Model file for the job. Use its own axes, mm. Round coordinates to 2 decimals unless told otherwise and drop trailing zeros. Order: outer loops, then holes, each group sorted by start corner. A loop starts at its lowest first (then second) coordinate and runs counter-clockwise, first axis right, second up. Notation, with made-up numbers: (60, -2.75) - (79, -2.75) arc R9 cw to (79, 1.25) - close; hole circle Ø4 at (62, 83.25). An arc over 180 degrees is marked (long way). Put each result on its own line as item: value. Start each with the question number.
Item 1: Saw through at A-A on z = 41. List the corners of the cut face in (x, y).
Item 2: Probe probe 1 along Y at (x, z) = (36.5, 70); probe 2 along Z at (x, y) = (-7.5, 9.5). List the from-to ranges inside material, lowest first.
Item 3: Saw through at B-B on x = -29.5. List the corners of the cut face in (y, z).
```python
from build123d import *

# Parameters (mm, degrees)
SZKIC1_W                    = 100
SZKIC1_H                    = 100
DODANIE_WYCI_GNI_CIE1_DEPTH = 100
SKORUPA2_T                  = 10


with BuildPart() as part:
    # Szkic1 → Dodanie-wyciągnięcie1 (new body)
    with BuildSketch(Plane.XY):
        Rectangle(SZKIC1_W, SZKIC1_H)
    extrude(amount=DODANIE_WYCI_GNI_CIE1_DEPTH)

    # Skorupa2 (no face opened: a closed hollow body)
    add(offset(amount=-SKORUPA2_T, mode=Mode.PRIVATE), mode=Mode.SUBTRACT)


solid = part.part
```
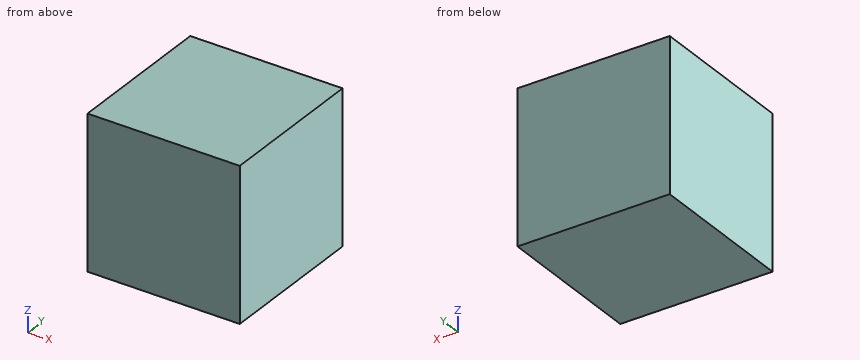
Results found:
1. outline: (-50, -50) - (50, -50) - (50, 50) - (-50, 50) - close; hole (-40, -40) - (40, -40) - (40, 40) - (-40, 40) - close
2. probe 1: y = -50 to -40, 40 to 50
2. probe 2: z = 0 to 10, 90 to 100
3. outline: (-50, 0) - (50, 0) - (50, 100) - (-50, 100) - close; hole (-40, 10) - (40, 10) - (40, 90) - (-40, 90) - close
